```python
from build123d import *

# Parameters (mm, degrees)
BOSS_EXTRUDE1_START = 12
SKETCH1_R           = 4
BOSS_EXTRUDE1_DEPTH = 4
BOSS_EXTRUDE2_START = -12
SKETCH1_2_R         = 4
BOSS_EXTRUDE2_DEPTH = 4
SKETCH2_W           = 30
SKETCH2_H           = 32
BOSS_EXTRUDE3_DEPTH = 4
SKETCH3_W           = 48
SKETCH3_H           = 32
BOSS_EXTRUDE4_DEPTH = 3
SKETCH3_3_W         = 4
SKETCH3_3_H         = 32
BOSS_EXTRUDE5_DEPTH = 30
SKETCH4_R           = 3
CUT_EXTRUDE1_DEPTH  = 78.723870207


with BuildPart() as part:
    # Sketch1 → Boss-Extrude1 (new body)
    with BuildSketch(Plane(origin=(0, 0, 0), x_dir=(1, 0, 0), z_dir=(0, 1, 0)).offset(BOSS_EXTRUDE1_START)):
        with BuildLine():
            Line((-15, 0), (-15, -25))
            Line((-15, -25), (15, -25))
            Line((15, -25), (15, 0))
            ThreePointArc((15, 0), (0, 15), (-15, 0))
        make_face()
        with Locations(Location((0, 0, 0), (0, 0, 270))):
            Circle(SKETCH1_R, mode=Mode.SUBTRACT)
    extrude(amount=BOSS_EXTRUDE1_DEPTH)



with BuildPart() as body_2:
    # Sketch1<2> → Boss-Extrude2 (new body)
    with BuildSketch(Plane(origin=(0, 0, 0), x_dir=(1, 0, 0), z_dir=(0, 1, 0)).offset(BOSS_EXTRUDE2_START)):
        with BuildLine():
            Line((-15, 0), (-15, -25))
            Line((-15, -25), (15, -25))
            Line((15, -25), (15, 0))
            ThreePointArc((15, 0), (0, 15), (-15, 0))
        make_face()
        with Locations(Location((0, 0, 0), (0, 0, 270))):
            Circle(SKETCH1_2_R, mode=Mode.SUBTRACT)
    extrude(amount=-BOSS_EXTRUDE2_DEPTH)


with BuildPart() as part_1:
    add(part.part)

    add(body_2.part)  # Boss-Extrude3 merges body 2
    # Sketch2 → Boss-Extrude3 (add)
    with BuildSketch(Plane.XY.offset(25)):
        Rectangle(SKETCH2_W, SKETCH2_H)
    extrude(amount=BOSS_EXTRUDE3_DEPTH)

    # Sketch3 → Boss-Extrude4 (add)
    with BuildSketch(Plane.XY.offset(29)):
        Rectangle(SKETCH3_W, SKETCH3_H)
    extrude(amount=BOSS_EXTRUDE4_DEPTH)

    # Sketch3<3> → Boss-Extrude5 (add)
    with BuildSketch(Plane.XY.offset(29)):
        with Locations((22, 0)):
            Rectangle(SKETCH3_3_W, SKETCH3_3_H)
        with Locations((-22, 0)):
            Rectangle(SKETCH3_3_W, SKETCH3_3_H)
    extrude(amount=BOSS_EXTRUDE5_DEPTH)

    # Sketch4 → Cut-Extrude1 (cut, through all)
    with BuildSketch(Plane(origin=(-24, 0, 0), x_dir=(0, -1, 0), z_dir=(1, 0, 0))):
        with BuildLine():
            Line((16, -59), (16, -43))
            ThreePointArc((16, -43), (11.313708499, -54.313708499), (0, -59))
            Line((0, -59), (16, -59))
        make_face()
        with Locations((0, -43)):
            Circle(SKETCH4_R)
        with BuildLine():
            Line((-16, -59), (0, -59))
            ThreePointArc((0, -59), (-11.313708499, -54.313708499), (-16, -43))
            Line((-16, -43), (-16, -59))
        make_face()
    extrude(amount=CUT_EXTRUDE1_DEPTH, mode=Mode.SUBTRACT)


solid = part_1.part
```
Read the model definition and answer for the solid it produces. Units are mm, in the model's axes. A direction names the side the tool comes from. Give positions to 0.01 mm unless a question says otherwise; leave off trailing zeros. Loops run counter-clockwise (first coordinate to the right, second up) from the corner with the lowest first, then second, coordinate; pieces in that order, holes last.
Item 1: Find the intervals of material crossed by line 1 along X through (y, z) = (-8, 38); line 2 along X through (y, z) = (-13.75, 0); line 3 along Z through (x, y) = (21.45, 0), in increasing order.
Item 2: Each of these flat-tipped pins is pushed along its axis until it touches: pin 1 Ø7 at (x, y) = (-21, -2) entering from -Z; pin 2 Ø3 at (x, y) = (-15, -1.5) entering from -Z; pin 3 Ø19 at (x, y) = (-3.5, -3) entering from -Z. Where does it stop, or does it pass through?
Item 3: The part is cut by section A-A (z = 12). Write down the section's boundary in (x, y).
Item 4: The part is cut by section B-B (x = 0). Write down the section's boundary in (y, z).
Item 5: The mould has two halves that part along Z. Classify faces 5 (the cylindrical face through (-22, 0, 40)), 6 (the flat face through (15, 2.3, 25.2)), 7 (the flat face through (0, 0, 25)): released by +Z, released by -Z, zero draft, split by the parting line, or undercut.
Item 6: The part is cut by section D-D (x = 21). Write down the section's boundary in (y, z).
Item 7: The part is cut by section C-C (y = 13). Write down the section's boundary in (x, z), and give its area (3 significant figures).
Item 8: For faces 1 (the flat face through (-20, 0, 29)), 2 (the flat face through (0, 0, 32)), 3 (the flat face through (19, 0, 29)), 4 (the flat face through (0, 12, 5)), determine the directions among +Z, -Z, +X, -X, +Y, -Y from which every point of the face is accessible in a straight line to the end or side of a thin tool.
Taken from the geometry:
1. line 1: x = -24 to -20, 20 to 24
1. line 2: x = -15 to -4, 4 to 15
1. line 3: z = 29 to 40, 46 to 59
2. pin 1: stops at z = 29
2. pin 2: stops at z = 25
2. pin 3: stops at z = -14.99
3. outline: (-15, -16) - (15, -16) - (15, -12) - (-15, -12) - close; (-15, 12) - (15, 12) - (15, 16) - (-15, 16) - close
4. outline: (-16, -15) - (-12, -15) - (-12, -4) - (-16, -4) - close; (-16, 4) - (-12, 4) - (-12, 25) - (12, 25) - (12, 4) - (16, 4) - (16, 32) - (-16, 32) - close; (12, -15) - (16, -15) - (16, -4) - (12, -4) - close
5. face 5: undercut
5. face 6: zero draft
5. face 7: released by -Z
6. outline: (-16, 29) - (16, 29) - (16, 43) arc R16 ccw to (-16, 43) - close; hole circle Ø6 at (0, 43)
7. outline: (-24, 29) - (-15, 29) - (-15, 0) arc R15 ccw to (15, 0) - (15, 29) - (24, 29) - (24, 52.33) - (20, 52.33) - (20, 32) - (-20, 32) - (-20, 52.33) - (-24, 52.33) - close; hole circle Ø8 at (0, 0)
7. area: 1,480 mm2
8. face 1: -Z, -X, +Y, -Y
8. face 2: +Z, +Y, -Y
8. face 3: -Z, +X, +Y, -Y
8. face 4: -Z, +X, -X
